Here's the drawing with two shaded views (mm, measured from the low corner). I have some questions. A direction names the side the tool comes from. Coordinates: 2 decimals unless noted, no trailing zeros. Loops run counter-clockwise (first coordinate to the right, second up) from the corner with the lowest first, then second, coordinate; pieces in that order, holes last. Notation, with made-up numbers: (44, 45.25) -> (58, 45.25) arc R31 cw to (58, 69.25) -> close; hole circle Ø5 at (60, -22). An arc over 180 degrees is marked (long way). Use CSV: the item, a comma, the result in double quotes. Start each with the question number.
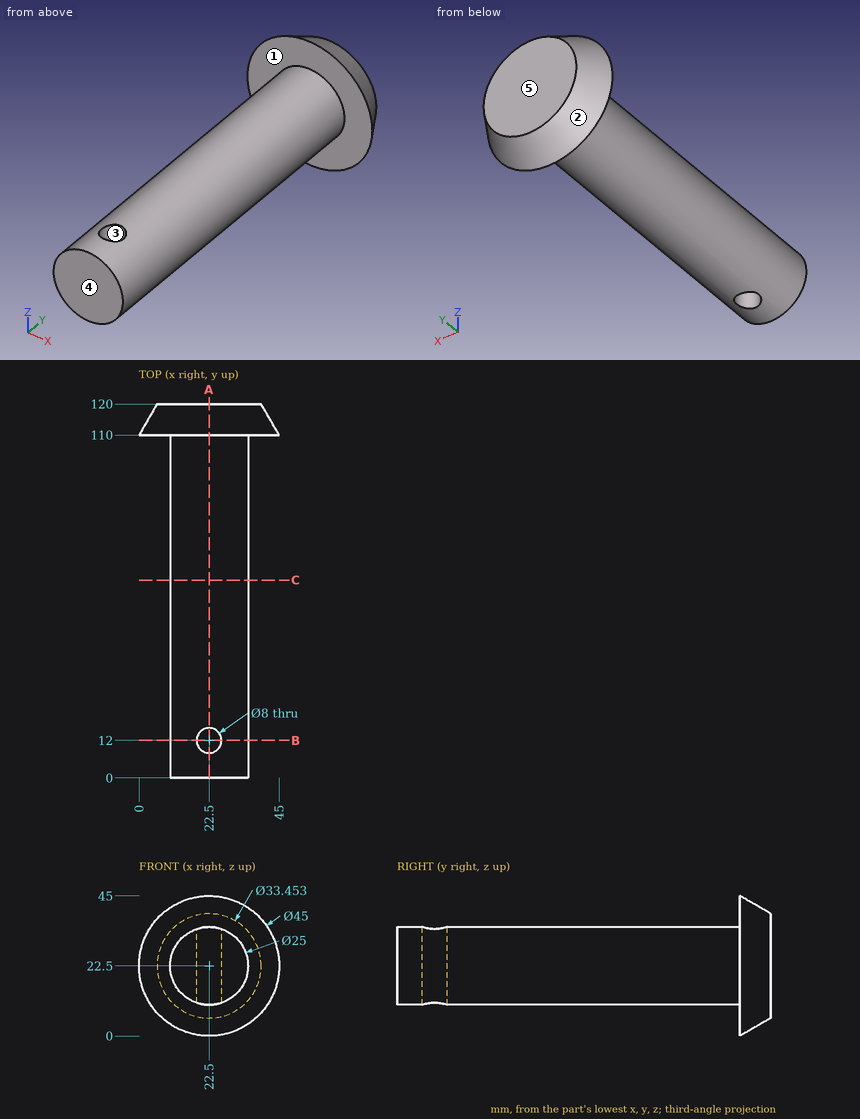
1) Please list where these lines run through material, in increasing order: L1, parallel to X at y = 12, z = 22; L2, parallel to Y at x = 29.5, z = 9; L3, parallel to X at y = 9, z = 23.5. Write a range as [from, to].
2) For P1, Ø10.5, axis at x = 22.5, y = 12, coming from the +Z side; P2, Ø1, axis at x = 36, z = 10.5, coming from the +Y side; P3, Ø10, axis at x = 21.5, z = 5, coming from the +Y side; P4, Ø8, axis at y = 87.5, z = 16.5, coming from the +X side, each with a flat end and sliding along its axis, tell me the tip position at first contact or that it passes through.
3) I want a section at A-A, the plane x = 22.5. Please give me the cut outline in (y, z).
4) Which directions (+Z, -Z, +X, -X, +Y, -Y) give clear straight access to the entire face, cutting with the end or side of a thin tool? Please do the marked faces 1 and 2.
5) I want a section at C-C, the plane y = 63.5. Please give me the cut outline in (x, z), plus the area to 3 significant figures.
6) Thinking about a two-plate mould opening in Y: for the marked faces 3, 4 and 5, which applies, pulls with the +Y half, pulls with the -Y half, needs draft (parallel to the pull), parting line crosses it, or undercut?
7) I want a section at B-B, the plane y = 12. Please give me the cut outline in (x, z).
Return value:
1,L1,"x = [10.01, 18.5], [26.5, 34.99]"
1,L2,"y = [110, 120]"
1,L3,"x = [10.04, 19.85], [25.15, 34.96]"
2,P1,"stops at z = 35"
2,P2,"stops at y = 118.55"
2,P3,"stops at y = 120"
2,P4,"stops at x = 34.84"
3,outline,"(0, 10) -> (8, 10) -> (8, 35) -> (0, 35) -> close; (16, 10) -> (110, 10) -> (110, 0) -> (120, 5.77) -> (120, 39.23) -> (110, 45) -> (110, 35) -> (16, 35) -> close"
4,face 1,"-Y"
4,face 2,"+Y"
5,outline,"circle Ø25 at (22.5, 22.5)"
5,area,"491 mm²"
6,face 3,"undercut"
6,face 4,"pulls with the -Y half"
6,face 5,"pulls with the +Y half"
7,outline,"(18.5, 10.66) -> (18.5, 34.34) arc R12.5 ccw to start; (26.5, 10.66) arc R12.5 ccw to (26.5, 34.34) -> close"
